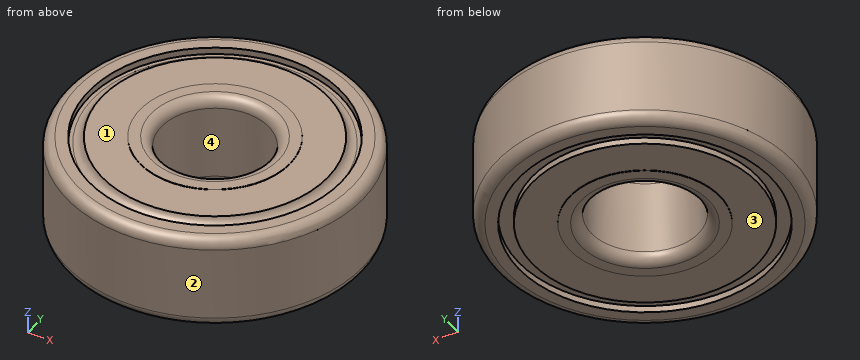
```python
from build123d import *


with BuildPart() as part:
    # Sketch1 → Revolve1 (revolve)
    with BuildSketch(Plane(origin=(0, 0, 0), x_dir=(1, 0, 0), z_dir=(0, 1, 0))):
        with BuildLine():
            Line((4.0005, 2.7305), (4.0005, -2.7305))
            ThreePointArc((4.0005, -2.7305), (4.223684633, -3.269315367), (4.7625, -3.4925))
            Line((4.7625, -3.4925), (5.588, -3.4925))
            Line((5.588, -3.4925), (5.588, -3.4671))
            Line((5.588, -3.4671), (8.3947, -3.4671))
            ThreePointArc((8.3947, -3.4671), (8.674827163, -3.116600484), (9.103628515, -2.9845))
            Line((9.103628515, -2.9845), (9.398, -2.9845))
            Line((9.398, -2.9845), (9.398, -3.4925))
            Line((9.398, -3.4925), (10.2489, -3.4925))
            ThreePointArc((10.2489, -3.4925), (10.787715367, -3.269315367), (11.0109, -2.7305))
            Line((11.0109, -2.7305), (11.0109, 2.7305))
            ThreePointArc((11.0109, 2.7305), (10.787715367, 3.269315367), (10.2489, 3.4925))
            Line((10.2489, 3.4925), (9.398, 3.4925))
            Line((9.398, 3.4925), (9.398, 2.9845))
            Line((9.398, 2.9845), (8.3947, 2.9845))
            Line((8.3947, 2.9845), (8.3947, 3.4671))
            Line((8.3947, 3.4671), (5.588, 3.4671))
            Line((5.588, 3.4671), (5.588, 3.4925))
            Line((5.588, 3.4925), (4.7625, 3.4925))
            ThreePointArc((4.7625, 3.4925), (4.223684633, 3.269315367), (4.0005, 2.7305))
        make_face()
    revolve(axis=Axis((0, 0, -3.495313106), (0, 0, 1)))


solid = part.part
```
Can you work these out from the model? Positions are in its coordinate system, mm. Face numbers are marked on the shaded views. A direction names the side the tool comes from. Round coordinates to 2 decimals unless told otherwise and drop trailing zeros. Loops run counter-clockwise (first coordinate to the right, second up) from the corner with the lowest first, then second, coordinate; pieces in that order, holes last. Notation, with made-up numbers: (-4, 16) -> (42, 16) arc R11 ccw to (42, 23) -> close; hole circle Ø1 at (82.25, -36.5). An arc over 180 degrees is marked (long way). One line per item, written item: value. Start each with the question number.
1. If I drill on probe 1 along Y at (x, z) = (0, 3.35); probe 2 along Y at (x, z) = (0, -3.3); probe 3 along Y at (x, z) = (3.5, -1), over which ranges is the centre line in solid material (lowest first)?
2. For pin 1 (5 mm diameter, centred on x = 0, y = 0, fed in from -Z); pin 2 (3 mm diameter, centred on y = 5, z = -0.5, fed in from +X); pin 3 (1 mm diameter, centred on x = -5, z = -1, fed in from +Y); pin 4 (8.5 mm diameter, centred on x = 0, y = 3.5, fed in from +Z), each with a flat end and sliding along its axis, tell me the tip position at first contact or that it passes through.
3. If we mould it in two halves opening along Y, with no side actions, what happens to the marked faces 1 and 2? For each: pulls with the +Y half, pulls with the -Y half, needs draft (parallel to the pull), parting line crosses it, or undercut.
4. If we section it at A-A, the plane z = 0.5: Write out the boundary of the cut face in (x, y), then the cut area to 3 significant figures.
5. For the marked faces 3 and 4, which set-ups out of +Z, -Z, +X, -X, +Y, -Y let a thin tool reach every point of the face, with its end or its side?
Calculated:
1. probe 1: y = -10.69 to -9.4, -8.45 to -4.32, 4.32 to 8.45, 9.4 to 10.69
1. probe 2: y = -10.76 to -9.4, -8.39 to -4.26, 4.26 to 8.39, 9.4 to 10.76
1. probe 3: y = -10.44 to -1.94, 1.94 to 10.44
2. pin 1: passes through
2. pin 2: stops at x = 10.44
2. pin 3: stops at y = 10.05
2. pin 4: stops at z = 3.49
3. face 1: undercut
3. face 2: parting line crosses it
4. outline: circle Ø22.02 at (0, 0); hole circle Ø8 at (0, 0)
4. area: 331 mm²
5. face 3: -Z
5. face 4: +Z, -Z
